```python
from build123d import *

# Parameters (mm, degrees)
SKETCH1_W           = 31.75
SKETCH1_H           = 63.5
SKETCH1_W_2         = 25.4
SKETCH1_H_2         = 57.15
BOSS_EXTRUDE1_DEPTH = 647.7
CUT_EXTRUDE1_REACH  = 653.339
SKETCH3_W           = 50.8
SKETCH3_H           = 25.4
CUT_EXTRUDE2_REACH  = 653.339
SKETCH6_R           = 15.5575
SKETCH6_R_2         = 3.175
CUT_EXTRUDE3_REACH  = 653.339
SKETCH7_R           = 6.35
SKETCH8_R           = 3.175
CUT_EXTRUDE4_DEPTH  = 652.099933119
CUT_EXTRUDE5_REACH  = 653.1
SKETCH9_R           = 1.8415


with BuildPart() as part:
    # Sketch1 → Boss-Extrude1 (new body)
    with BuildSketch(Plane.XY):
        with Locations((3.710272719, -29.23968021)):
            Rectangle(SKETCH1_W, SKETCH1_H)
        with Locations((3.710272719, -29.23968021)):
            Rectangle(SKETCH1_W_2, SKETCH1_H_2, mode=Mode.SUBTRACT)
    extrude(amount=BOSS_EXTRUDE1_DEPTH)

    # Cut-Extrude1: up to this face of the body (flat: up to its plane)
    cut_extrude1_end = Plane(part.part.faces().sort_by_distance((19.585272719, -29.23968021, 323.85))[0])
    # Sketch3 → Cut-Extrude1 (cut, up to the picked face)
    with BuildSketch(Plane.ZY.offset(12.164727281), mode=Mode.PRIVATE) as cut_extrude1_sk1:
        with BuildLine():
            Line((31.7754, -13.36468021), (120.6754, -13.36468021))
            ThreePointArc((120.6754, -13.36468021), (122.92046403, -14.294616179), (123.8504, -16.53968021))
            Line((123.8504, -16.53968021), (123.8504, -41.93968021))
            ThreePointArc((123.8504, -41.93968021), (122.92046403, -44.18474424), (120.6754, -45.11468021))
            Line((120.6754, -45.11468021), (31.7754, -45.11468021))
            ThreePointArc((31.7754, -45.11468021), (29.53033597, -44.18474424), (28.6004, -41.93968021))
            Line((28.6004, -41.93968021), (28.6004, -16.53968021))
            ThreePointArc((28.6004, -16.53968021), (29.53033597, -14.294616179), (31.7754, -13.36468021))
        make_face()
    cut_extrude1_tool1 = split(extrude(cut_extrude1_sk1.sketch, amount=-CUT_EXTRUDE1_REACH, mode=Mode.PRIVATE), bisect_by=cut_extrude1_end, keep=Keep.BOTH, mode=Mode.PRIVATE)
    # Sketch3 → Cut-Extrude1 (cut, up to the picked face)
    with BuildSketch(Plane.ZY.offset(12.164727281), mode=Mode.PRIVATE) as cut_extrude1_sk2:
        with BuildLine():
            ThreePointArc((619.0996, -41.93968021), (618.16966403, -44.18474424), (615.9246, -45.11468021))
            Line((615.9246, -45.11468021), (527.0246, -45.11468021))
            ThreePointArc((527.0246, -45.11468021), (524.77953597, -44.18474424), (523.8496, -41.93968021))
            Line((523.8496, -41.93968021), (523.8496, -16.53968021))
            ThreePointArc((523.8496, -16.53968021), (524.77953597, -14.294616179), (527.0246, -13.36468021))
            Line((527.0246, -13.36468021), (615.9246, -13.36468021))
            ThreePointArc((615.9246, -13.36468021), (618.16966403, -14.294616179), (619.0996, -16.53968021))
            Line((619.0996, -16.53968021), (619.0996, -41.93968021))
        make_face()
    cut_extrude1_tool2 = split(extrude(cut_extrude1_sk2.sketch, amount=-CUT_EXTRUDE1_REACH, mode=Mode.PRIVATE), bisect_by=cut_extrude1_end, keep=Keep.BOTH, mode=Mode.PRIVATE)
    # Sketch3 → Cut-Extrude1 (cut, up to the picked face)
    with BuildSketch(Plane.ZY.offset(12.164727281), mode=Mode.PRIVATE) as cut_extrude1_sk3:
        with Locations((196.85, -48.28968021)):
            Rectangle(SKETCH3_W, SKETCH3_H)
    cut_extrude1_tool3 = split(extrude(cut_extrude1_sk3.sketch, amount=-CUT_EXTRUDE1_REACH, mode=Mode.PRIVATE), bisect_by=cut_extrude1_end, keep=Keep.BOTH, mode=Mode.PRIVATE)
    # Sketch3 → Cut-Extrude1 (cut, up to the picked face)
    with BuildSketch(Plane.ZY.offset(12.164727281), mode=Mode.PRIVATE) as cut_extrude1_sk4:
        with Locations((450.85, -48.28968021)):
            Rectangle(SKETCH3_W, SKETCH3_H)
    cut_extrude1_tool4 = split(extrude(cut_extrude1_sk4.sketch, amount=-CUT_EXTRUDE1_REACH, mode=Mode.PRIVATE), bisect_by=cut_extrude1_end, keep=Keep.BOTH, mode=Mode.PRIVATE)
    add(cut_extrude1_tool1.solids().sort_by(Axis((-12.164727, -29.23968, 76.2254), (1, 0, 0)))[0], mode=Mode.SUBTRACT)
    add(cut_extrude1_tool2.solids().sort_by(Axis((-12.164727, -29.23968, 571.4746), (1, 0, 0)))[0], mode=Mode.SUBTRACT)
    add(cut_extrude1_tool3.solids().sort_by(Axis((-12.164727, -48.28968, 196.85), (1, 0, 0)))[0], mode=Mode.SUBTRACT)
    add(cut_extrude1_tool4.solids().sort_by(Axis((-12.164727, -48.28968, 450.85), (1, 0, 0)))[0], mode=Mode.SUBTRACT)

    # Cut-Extrude2: up to this face of the body (flat: up to its plane)
    cut_extrude2_end = Plane(part.part.faces().sort_by_distance((-12.164727281, -27.727830199, 323.85))[0])
    # Sketch6 → Cut-Extrude2 (cut, up to the picked face)
    with BuildSketch(Plane(origin=(19.585272719, 0, 0), x_dir=(0, 0, -1), z_dir=(1, 0, 0)), mode=Mode.PRIVATE) as cut_extrude2_sk1:
        with Locations(Location((-323.85, -34.00218021, 0), (0, 0, 90))):
            Circle(SKETCH6_R)
    cut_extrude2_tool1 = split(extrude(cut_extrude2_sk1.sketch, amount=-CUT_EXTRUDE2_REACH, mode=Mode.PRIVATE), bisect_by=cut_extrude2_end, keep=Keep.BOTH, mode=Mode.PRIVATE)
    # Sketch6 → Cut-Extrude2 (cut, up to the picked face)
    with BuildSketch(Plane(origin=(19.585272719, 0, 0), x_dir=(0, 0, -1), z_dir=(1, 0, 0)), mode=Mode.PRIVATE) as cut_extrude2_sk2:
        with Locations(Location((-273.05, -34.00218021, 0), (0, 0, 90))):
            Circle(SKETCH6_R)
    cut_extrude2_tool2 = split(extrude(cut_extrude2_sk2.sketch, amount=-CUT_EXTRUDE2_REACH, mode=Mode.PRIVATE), bisect_by=cut_extrude2_end, keep=Keep.BOTH, mode=Mode.PRIVATE)
    # Sketch6 → Cut-Extrude2 (cut, up to the picked face)
    with BuildSketch(Plane(origin=(19.585272719, 0, 0), x_dir=(0, 0, -1), z_dir=(1, 0, 0)), mode=Mode.PRIVATE) as cut_extrude2_sk3:
        with Locations(Location((-365.125, -7.01468021, 0), (0, 0, 90))):
            Circle(SKETCH6_R_2)
    cut_extrude2_tool3 = split(extrude(cut_extrude2_sk3.sketch, amount=-CUT_EXTRUDE2_REACH, mode=Mode.PRIVATE), bisect_by=cut_extrude2_end, keep=Keep.BOTH, mode=Mode.PRIVATE)
    # Sketch6 → Cut-Extrude2 (cut, up to the picked face)
    with BuildSketch(Plane(origin=(19.585272719, 0, 0), x_dir=(0, 0, -1), z_dir=(1, 0, 0)), mode=Mode.PRIVATE) as cut_extrude2_sk4:
        with Locations(Location((-231.775, -7.01468021, 0), (0, 0, 90))):
            Circle(SKETCH6_R_2)
    cut_extrude2_tool4 = split(extrude(cut_extrude2_sk4.sketch, amount=-CUT_EXTRUDE2_REACH, mode=Mode.PRIVATE), bisect_by=cut_extrude2_end, keep=Keep.BOTH, mode=Mode.PRIVATE)
    # Sketch6 → Cut-Extrude2 (cut, up to the picked face)
    with BuildSketch(Plane(origin=(19.585272719, 0, 0), x_dir=(0, 0, -1), z_dir=(1, 0, 0)), mode=Mode.PRIVATE) as cut_extrude2_sk5:
        with Locations(Location((-365.125, -51.46468021, 0), (0, 0, 90))):
            Circle(SKETCH6_R_2)
    cut_extrude2_tool5 = split(extrude(cut_extrude2_sk5.sketch, amount=-CUT_EXTRUDE2_REACH, mode=Mode.PRIVATE), bisect_by=cut_extrude2_end, keep=Keep.BOTH, mode=Mode.PRIVATE)
    # Sketch6 → Cut-Extrude2 (cut, up to the picked face)
    with BuildSketch(Plane(origin=(19.585272719, 0, 0), x_dir=(0, 0, -1), z_dir=(1, 0, 0)), mode=Mode.PRIVATE) as cut_extrude2_sk6:
        with Locations(Location((-231.775, -51.46468021, 0), (0, 0, 90))):
            Circle(SKETCH6_R_2)
    cut_extrude2_tool6 = split(extrude(cut_extrude2_sk6.sketch, amount=-CUT_EXTRUDE2_REACH, mode=Mode.PRIVATE), bisect_by=cut_extrude2_end, keep=Keep.BOTH, mode=Mode.PRIVATE)
    add(cut_extrude2_tool1.solids().sort_by(Axis((19.585273, -34.00218, 323.85), (-1, 0, 0)))[0], mode=Mode.SUBTRACT)
    add(cut_extrude2_tool2.solids().sort_by(Axis((19.585273, -34.00218, 273.05), (-1, 0, 0)))[0], mode=Mode.SUBTRACT)
    add(cut_extrude2_tool3.solids().sort_by(Axis((19.585273, -7.01468, 365.125), (-1, 0, 0)))[0], mode=Mode.SUBTRACT)
    add(cut_extrude2_tool4.solids().sort_by(Axis((19.585273, -7.01468, 231.775), (-1, 0, 0)))[0], mode=Mode.SUBTRACT)
    add(cut_extrude2_tool5.solids().sort_by(Axis((19.585273, -51.46468, 365.125), (-1, 0, 0)))[0], mode=Mode.SUBTRACT)
    add(cut_extrude2_tool6.solids().sort_by(Axis((19.585273, -51.46468, 231.775), (-1, 0, 0)))[0], mode=Mode.SUBTRACT)

    # Sketch7 → Cut-Extrude3 (cut, up to next)
    with BuildSketch(Plane(origin=(19.585272719, 0, 0), x_dir=(0, 0, -1), z_dir=(1, 0, 0)), mode=Mode.PRIVATE) as cut_extrude3_sk1:
        with Locations(Location((-365.125, -7.01468021, 0), (0, 0, 90))):
            Circle(SKETCH7_R)
    cut_extrude3_tool1 = extrude(cut_extrude3_sk1.sketch, amount=-CUT_EXTRUDE3_REACH, mode=Mode.PRIVATE) & part.part
    # Sketch7 → Cut-Extrude3 (cut, up to next)
    with BuildSketch(Plane(origin=(19.585272719, 0, 0), x_dir=(0, 0, -1), z_dir=(1, 0, 0)), mode=Mode.PRIVATE) as cut_extrude3_sk2:
        with Locations(Location((-365.125, -51.46468021, 0), (0, 0, 90))):
            Circle(SKETCH7_R)
    cut_extrude3_tool2 = extrude(cut_extrude3_sk2.sketch, amount=-CUT_EXTRUDE3_REACH, mode=Mode.PRIVATE) & part.part
    # Sketch7 → Cut-Extrude3 (cut, up to next)
    with BuildSketch(Plane(origin=(19.585272719, 0, 0), x_dir=(0, 0, -1), z_dir=(1, 0, 0)), mode=Mode.PRIVATE) as cut_extrude3_sk3:
        with Locations(Location((-231.775, -51.46468021, 0), (0, 0, 90))):
            Circle(SKETCH7_R)
    cut_extrude3_tool3 = extrude(cut_extrude3_sk3.sketch, amount=-CUT_EXTRUDE3_REACH, mode=Mode.PRIVATE) & part.part
    # Sketch7 → Cut-Extrude3 (cut, up to next)
    with BuildSketch(Plane(origin=(19.585272719, 0, 0), x_dir=(0, 0, -1), z_dir=(1, 0, 0)), mode=Mode.PRIVATE) as cut_extrude3_sk4:
        with Locations(Location((-231.775, -7.01468021, 0), (0, 0, 90))):
            Circle(SKETCH7_R)
    cut_extrude3_tool4 = extrude(cut_extrude3_sk4.sketch, amount=-CUT_EXTRUDE3_REACH, mode=Mode.PRIVATE) & part.part
    add(cut_extrude3_tool1.solids().sort_by_distance((19.585273, -7.01468, 365.125))[0], mode=Mode.SUBTRACT)
    add(cut_extrude3_tool2.solids().sort_by_distance((19.585273, -51.46468, 365.125))[0], mode=Mode.SUBTRACT)
    add(cut_extrude3_tool3.solids().sort_by_distance((19.585273, -51.46468, 231.775))[0], mode=Mode.SUBTRACT)
    add(cut_extrude3_tool4.solids().sort_by_distance((19.585273, -7.01468, 231.775))[0], mode=Mode.SUBTRACT)

    # Sketch8 → Cut-Extrude4 (cut, through all)
    with BuildSketch(Plane(origin=(0, 2.51031979, 0), x_dir=(1, 0, 0), z_dir=(0, 1, 0))):
        with Locations(Location((3.710272719, -184.15, 0), (0, 0, 180))):
            Circle(SKETCH8_R)
        with Locations(Location((3.710272719, -209.55, 0), (0, 0, 180))):
            Circle(SKETCH8_R)
        with Locations(Location((3.710272719, -438.15, 0), (0, 0, 90))):
            Circle(SKETCH8_R)
        with Locations(Location((3.710272719, -463.55, 0), (0, 0, 90))):
            Circle(SKETCH8_R)
    extrude(amount=-CUT_EXTRUDE4_DEPTH, mode=Mode.SUBTRACT)

    # Cut-Extrude5: up to this face of the body (flat: up to its plane)
    cut_extrude5_end = Plane(part.part.faces().sort_by_distance((3.710272719, -60.98968021, 561.975))[0])
    # Sketch9 → Cut-Extrude5 (cut, up to the picked face)
    with BuildSketch(Plane(origin=(0, 2.51031979, 0), x_dir=(1, 0, 0), z_dir=(0, 1, 0)), mode=Mode.PRIVATE) as cut_extrude5_sk1:
        with Locations(Location((3.710272719, -639.7625, 0), (0, 0, 180))):
            Circle(SKETCH9_R)
    cut_extrude5_tool1 = split(extrude(cut_extrude5_sk1.sketch, amount=-CUT_EXTRUDE5_REACH, mode=Mode.PRIVATE), bisect_by=cut_extrude5_end, keep=Keep.BOTH, mode=Mode.PRIVATE)
    # Sketch9 → Cut-Extrude5 (cut, up to the picked face)
    with BuildSketch(Plane(origin=(0, 2.51031979, 0), x_dir=(1, 0, 0), z_dir=(0, 1, 0)), mode=Mode.PRIVATE) as cut_extrude5_sk2:
        with Locations(Location((3.710272719, -7.9375, 0), (0, 0, 180))):
            Circle(SKETCH9_R)
    cut_extrude5_tool2 = split(extrude(cut_extrude5_sk2.sketch, amount=-CUT_EXTRUDE5_REACH, mode=Mode.PRIVATE), bisect_by=cut_extrude5_end, keep=Keep.BOTH, mode=Mode.PRIVATE)
    add(cut_extrude5_tool1.solids().sort_by(Axis((3.710273, 2.51032, 639.7625), (0, -1, 0)))[0], mode=Mode.SUBTRACT)
    add(cut_extrude5_tool2.solids().sort_by(Axis((3.710273, 2.51032, 7.9375), (0, -1, 0)))[0], mode=Mode.SUBTRACT)


solid = part.part
```
Check sheet for the modelled part. Datum: model origin and axes. Units: mm. A direction names the side the tool comes from. Round coordinates to 2 decimals unless told otherwise and drop trailing zeros. Order: outer loops, then holes, each group sorted by start corner. A loop starts at its lowest first (then second) coordinate and runs counter-clockwise, first axis right, second up. Notation, with made-up numbers: (83.5, 60) - (104.5, 60) arc R25 ccw to (104.5, 76) - close; hole circle Ø9 at (69.25, 80.25). An arc over 180 degrees is marked (long way). Answer as CSV lines item,"result". Start each with the question number.
1) Section check C-C (z = 273.05). Record the cut outline in (x, y), then the cut area to 3 significant figures.
2) Section check A-A (z = 84.5). Record the cut outline in (x, y).
3) Scan lines: probe 1 along Y at (x, z) = (2, 262.5); probe 2 along X at (y, z) = (-14, 451); probe 3 along Y at (x, z) = (17, 323). Record each from-to range of solid material in increasing order.
4) Depth check by flat-ended pin: pin 1 (5 mm diameter, centred on x = 6, z = 177, fed in from -Y); pin 2 (7.5 mm diameter, centred on y = -51.46, z = 231.78, fed in from +X). Enter the tip coordinate at first touch or a pass-through.
5) Section check B-B (z = 161.5). Record the cut outline in (x, y).
6) Tool access check on faces 1 (the face through (4, -59, 425.45)), 2 (the face through (4, -57.815, 561)), 3 (the face through (18.02, -8.391, 225.576)). Record the directions out of +Z, -Z, +X, -X, +Y, -Y that give a thin tool (end or side, any length) a straight path to the whole face; none if there is none.
7) Draft check along Y on faces 4 (the face through (18.02, -56.504, 227.911)), 5 (the face through (3, -60.99, 85)), 6 (the face through (16.41, -17, 319)), 7 (the face through (19.585, -16, 319)). Enter one of: +Y half, -Y half, draft (parallel to the pull), parting line (faces both ways), or undercut.
Determined:
1,outline,"(-12.16, -60.99) - (19.59, -60.99) - (19.59, -49.56) - (16.41, -49.56) - (16.41, -57.81) - (-8.99, -57.81) - (-8.99, -49.56) - (-12.16, -49.56) - close; (-12.16, -18.44) - (-8.99, -18.44) - (-8.99, -0.66) - (16.41, -0.66) - (16.41, -18.44) - (19.59, -18.44) - (19.59, 2.51) - (-12.16, 2.51) - close"
1,area,"367 mm^2"
2,outline,"(-12.16, -60.99) - (19.59, -60.99) - (19.59, -45.11) - (16.41, -45.11) - (16.41, -57.81) - (-8.99, -57.81) - (-8.99, -45.11) - (-12.16, -45.11) - close; (-12.16, -13.36) - (-8.99, -13.36) - (-8.99, -0.66) - (16.41, -0.66) - (16.41, -13.36) - (19.59, -13.36) - (19.59, 2.51) - (-12.16, 2.51) - close"
3,probe 1,"-60.99 to -57.81, -0.66 to 2.51"
3,probe 2,"-12.16 to -8.99, 16.41 to 19.59"
3,probe 3,"-60.99 to -49.54, -18.47 to 2.51"
4,pin 1,"y = -0.66"
4,pin 2,"x = -8.99"
5,outline,"(-12.16, -60.99) - (19.59, -60.99) - (19.59, 2.51) - (-12.16, 2.51) - close; hole (-8.99, -57.81) - (16.41, -57.81) - (16.41, -0.66) - (-8.99, -0.66) - close"
6,face 1,"+X, -X, -Y"
6,face 2,"+Z, -Z"
6,face 3,"+X"
7,face 4,"undercut"
7,face 5,"-Y half"
7,face 6,"undercut"
7,face 7,"draft"
